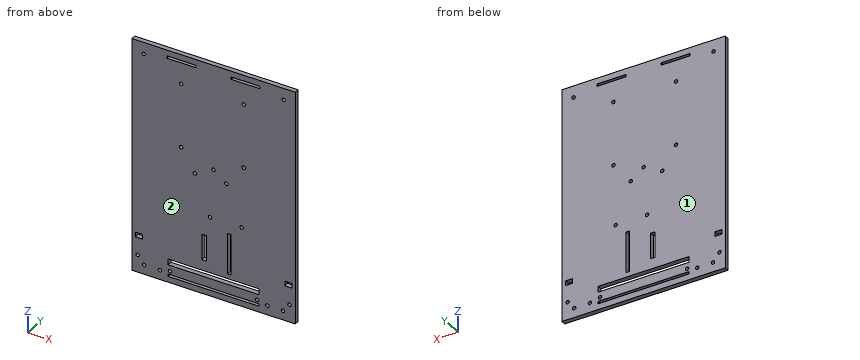
```python
from build123d import *

# Parameters (mm, degrees)
SKETCH1_W           = 140
SKETCH1_H           = 200
BOSS_EXTRUDE1_DEPTH = 4
SKETCH2_W           = 78
SKETCH2_H           = 2.05
SKETCH2_R           = 1.5
SKETCH2_H_2         = 5
CUT_EXTRUDE3_DEPTH  = 123.131077126
SKETCH3_W           = 6
SKETCH3_H           = 4
SKETCH3_R           = 1.5
CUT_EXTRUDE5_DEPTH  = 123.131077126
SKETCH4_R           = 1.5
CUT_EXTRUDE6_DEPTH  = 123.131077126
SKETCH6_W           = 3.05
SKETCH6_H           = 35
SKETCH6_W_2         = 4
SKETCH6_H_2         = 22
CUT_EXTRUDE13_DEPTH = 4
SKETCH7_R           = 1.5
CUT_EXTRUDE15_DEPTH = 123.131077126
SKETCH8_R           = 1.5
SKETCH8_W           = 25
SKETCH8_H           = 2.05
CUT_EXTRUDE16_DEPTH = 4


with BuildPart() as part:
    # Sketch1 → Boss-Extrude1 (new body)
    with BuildSketch(Plane(origin=(0, 0, 0), x_dir=(1, 0, 0), z_dir=(0, 1, 0))):
        Rectangle(SKETCH1_W, SKETCH1_H)
    extrude(amount=BOSS_EXTRUDE1_DEPTH)

    # Sketch2 → Cut-Extrude3 (cut, through all)
    with BuildSketch(Plane(origin=(0, 4, 0), x_dir=(1, 0, 0), z_dir=(0, 1, 0))):
        with Locations((0, 93.975)):
            Rectangle(SKETCH2_W, SKETCH2_H)
        with Locations(Location((-37.3, 90, 0), (0, 0, 270))):
            Circle(SKETCH2_R)
        with Locations(Location((37.3, 90, 0), (0, 0, 270))):
            Circle(SKETCH2_R)
        with Locations((0, 82.5)):
            Rectangle(SKETCH2_W, SKETCH2_H_2)
    extrude(amount=-CUT_EXTRUDE3_DEPTH, mode=Mode.SUBTRACT)

    # Sketch3 → Cut-Extrude5 (cut, through all)
    with BuildSketch(Plane(origin=(0, 4, 0), x_dir=(1, 0, 0), z_dir=(0, 1, 0))):
        with Locations((-64, 68)):
            Rectangle(SKETCH3_W, SKETCH3_H)
        with Locations(Location((65.055984274, 85, 0), (0, 0, 270))):
            Circle(SKETCH3_R)
        with Locations((64, 68)):
            Rectangle(SKETCH3_W, SKETCH3_H)
        with Locations(Location((-65.055984274, 85, 0), (0, 0, 270))):
            Circle(SKETCH3_R)
    extrude(amount=-CUT_EXTRUDE5_DEPTH, mode=Mode.SUBTRACT)

    # Sketch4 → Cut-Extrude6 (cut, through all)
    with BuildSketch(Plane(origin=(0, 4, 0), x_dir=(1, 0, 0), z_dir=(0, 1, 0))):
        with Locations(Location((59.5, 92, 0), (0, 0, 270))):
            Circle(SKETCH4_R)
        with Locations(Location((-59.5, 92, 0), (0, 0, 270))):
            Circle(SKETCH4_R)
        with Locations(Location((-46, 92, 0), (0, 0, 270))):
            Circle(SKETCH4_R)
        with Locations(Location((46, 92, 0), (0, 0, 90))):
            Circle(SKETCH4_R)
    extrude(amount=-CUT_EXTRUDE6_DEPTH, mode=Mode.SUBTRACT)

    # Sketch6 → Cut-Extrude13 (cut)
    with BuildSketch(Plane(origin=(0, 4, 0), x_dir=(1, 0, 0), z_dir=(0, 1, 0))):
        with Locations((13.525, 58.5)):
            Rectangle(SKETCH6_W, SKETCH6_H)
        with Locations((-8, 60)):
            Rectangle(SKETCH6_W_2, SKETCH6_H_2)
    extrude(amount=-CUT_EXTRUDE13_DEPTH, mode=Mode.SUBTRACT)

    # Sketch7 → Cut-Extrude15 (cut, through all)
    with BuildSketch(Plane(origin=(0, 4, 0), x_dir=(1, 0, 0), z_dir=(0, 1, 0))):
        with Locations(Location((25.802064663, -20.235830774, 0), (0, 0, 270))):
            Circle(SKETCH7_R)
        with Locations(Location((-27.802064663, -74.764169226, 0), (0, 0, 270))):
            Circle(SKETCH7_R)
        with Locations(Location((25.802064663, -74.764169226, 0), (0, 0, 270))):
            Circle(SKETCH7_R)
        with Locations(Location((24, 32, 0), (0, 0, 270))):
            Circle(SKETCH7_R)
        with Locations(Location((11, -1.5, 0), (0, 0, 270))):
            Circle(SKETCH7_R)
        with Locations(Location((-16, -1.5, 0), (0, 0, 270))):
            Circle(SKETCH7_R)
        with Locations(Location((-3, 32, 0), (0, 0, 270))):
            Circle(SKETCH7_R)
        with Locations(Location((-27.802064663, -20.235830774, 0), (0, 0, 270))):
            Circle(SKETCH7_R)
    extrude(amount=-CUT_EXTRUDE15_DEPTH, mode=Mode.SUBTRACT)

    # Sketch8 → Cut-Extrude16 (cut)
    with BuildSketch(Plane(origin=(0, 4, 0), x_dir=(1, 0, 0), z_dir=(0, 1, 0))):
        with Locations(Location((0, -10, 0), (0, 0, 270))):
            Circle(SKETCH8_R)
        with Locations(Location((-60, -90, 0), (0, 0, 270))):
            Circle(SKETCH8_R)
        with Locations(Location((60, -90, 0), (0, 0, 90))):
            Circle(SKETCH8_R)
        with Locations((27.5, -93.975)):
            Rectangle(SKETCH8_W, SKETCH8_H)
        with Locations((-27.5, -93.975)):
            Rectangle(SKETCH8_W, SKETCH8_H)
    extrude(amount=-CUT_EXTRUDE16_DEPTH, mode=Mode.SUBTRACT)


solid = part.part
```
Check sheet for the modelled part. Datum: model origin and axes. Units: mm. Face numbers are marked on the shaded views. Coordinates: 2 decimals unless noted, no trailing zeros. Order: outer loops, then holes, each group sorted by start corner. A loop starts at its lowest first (then second) coordinate and runs counter-clockwise, first axis right, second up. Notation, with made-up numbers: (21.5, -4.5) -> (47.5, -4.5) arc R20 ccw to (47.5, 7.5) -> close; hole circle Ø2 at (77.5, -14). An arc over 180 degrees is marked (long way). Write item = value, one per line. Start each with the question number.
1) Mould release check, pull along Y, two halves, no side actions. Record for the marked faces 1 and 2: +Y half, -Y half, draft (parallel to the pull), parting line (faces both ways), or undercut.
2) Go/stop test with a flat-tipped pin: P1, Ø5, axis at x = -12, z = -24.5, coming from the -Y side. Record where the tip stops, or that it passes through.
3) Material ranges on L1, parallel to X at y = 1.35, z = -92; L2, parallel to Z at x = 29, y = 0.25; L3, parallel to X at y = 0.75, z = 75, recorded low to high.
4) Cross-section at B-B (y = 2.35). State how many separate pieces and enclosed holes the cut face has, then the cut area to 3 significant figures.
5) Cross-section at A-A (x = 33). Enter the section's corners in (y, z), then the cut area to 3 significant figures.
Ans:
q1.face_1 = +Y half
q1.face_2 = -Y half
q2.P1 = 0
q3.L1 = -70 to -61, -58 to -47.5, -44.5 to 44.5, 47.5 to 58, 61 to 70
q3.L2 = -100 to -95, -92.95 to -85, -80 to 92.95, 95 to 100
q3.L3 = -70 to -29.28, -26.32 to 24.32, 27.28 to 70
q4.separate_pieces = 1
q4.enclosed_holes = 27
q4.area = 27,000 mm²
q5.outline = (0, -100) -> (4, -100) -> (4, -95) -> (0, -95) -> close; (0, -92.95) -> (4, -92.95) -> (4, -85) -> (0, -85) -> close; (0, -80) -> (4, -80) -> (4, 92.95) -> (0, 92.95) -> close; (0, 95) -> (4, 95) -> (4, 100) -> (0, 100) -> close
q5.area = 764 mm²
